Design review of the part built by this model. Coordinates are the model's own, in mm. Face numbers are marked on the shaded views. Give positions to 0.01 mm unless a question says otherwise; leave off trailing zeros. Loops run counter-clockwise (first coordinate to the right, second up) from the corner with the lowest first, then second, coordinate; pieces in that order, holes last.
Autodesk Inventor part; units mm, degrees
ref_plane "YZ Plane" through (0, 0, 0) normal (1, 0, 0) x (0, 1, 0)
ref_plane "XZ Plane" through (0, 0, 0) normal (0, 1, 0) x (-1, 0, 0)
ref_plane "XY Plane" through (0, 0, 0) normal (0, 0, 1) x (1, 0, 0)
sketch "Sketch1" plane through (0, 0, 0) normal (0, 0, 1) x (1, 0, 0)
  line L0 (0, 3) -> (3, 3)
  line L1 (6, 0) -> (6, 0)
  line L2 (3, -3) -> (0, -3)
  line L3 (0, -3) -> (0, 3)
  arc A0 (6, 0) -> (3, 3) centre (3, 0) ccw
  arc A1 (3, -3) -> (6, 0) centre (3, 0) ccw
  point P0 (0, 0)
  point P1 (0, 0)
  dimension "d0" = 3
  dimension "d1" = 6
  dimension "d2" = 6
extrude "Extrusion1" add sketch "Sketch1" along normal blind 6.5
sketch "Sketch2" plane through (0, -3, 0) normal (-1, 0, 0) x (0, 0, 1)
  line L0 (0, 6) -> (6.5, 6)
  line L1 (6.5, 6) -> (6.5, 0)
  line L2 (0, 0) -> (6.5, 0)
  line L3 (0, 0) -> (0, 6)
  line L4 (3.25, 6) -> (3.25, 0) construction
  line L5 (0, 3) -> (6.5, 3) construction
  point P0 (3.25, 3)
hole "Hole1" at (0, 0, 3.25) direction (1, 0, 0) diameter 3.2 depth 2
properties part number "Belt Tensioner" material "PC/ABS Plastic"
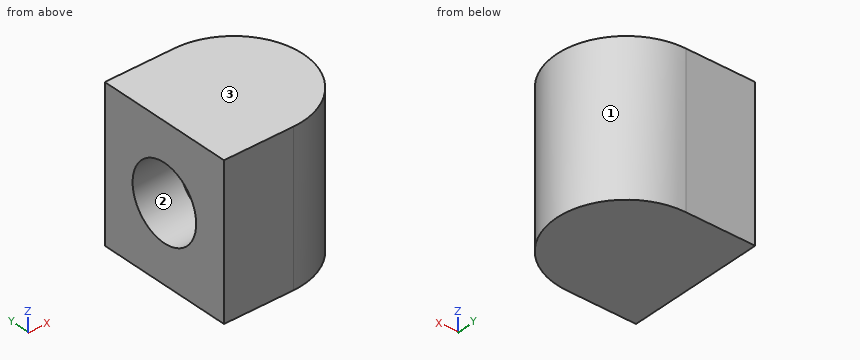
Q1. Take a section at B-B (z = 3.25). Give the boundary of the cut face in (x, y), plus the area to 3 significant figures.
Results:
outline: (0, -3) - (3, -3) arc R3 ccw to (3, 3) - (0, 3) - (0, 1.6) - (2, 1.6) - (2, -1.6) - (0, -1.6) - close
area: 25.7 mm2
Q2. Take a section at D-D (x = 3.9). Give the boundary of the cut face in (y, z).
Results:
outline: (-2.86, 0) - (2.86, 0) - (2.86, 6.5) - (-2.86, 6.5) - close
Q3. Draft analysis for pull direction Z (two halves, no side actions). For the marked faces 1, 2 and 3, state which applies: pulls with the +Z half, pulls with the -Z half, needs draft (parallel to the pull), parting line crosses it, or undercut.
Results:
face 1: needs draft
face 2: undercut
face 3: pulls with the +Z half
Q4. Take a section at C-C (y = 0). Give the boundary of the cut face in (x, z), plus the area to 3 significant figures.
Results:
outline: (0, 0) - (6, 0) - (6, 6.5) - (0, 6.5) - (0, 4.85) - (2, 4.85) - (2, 1.65) - (0, 1.65) - close
area: 32.6 mm2
Q5. Wall thickness on line 1 (Y direction, x = 1.55, z = 3.25); line 2 (Z direction, x = 1.55, y = 0); line 3 (Y direction, x = 1.6, z = 4.25): over which ranges is each line inside the solid? List them lowest first.
Results:
line 1: y = -3 to -1.6, 1.6 to 3
line 2: z = 0 to 1.65, 4.85 to 6.5
line 3: y = -3 to -1.25, 1.25 to 3
Q6. Insertion check: pin 1 (1 mm diameter, centred on x = 5.5, z = 5, fed in from -Y). The pin has a flat end and moves straight along its axis. Give the tip position at first contact, or say it passes through.
Results:
pin 1: stops at y = -2.24
Q7. Take a section at A-A (x = 1.85). Give the boundary of the cut face in (y, z).
Results:
outline: (-3, 0) - (3, 0) - (3, 6.5) - (-3, 6.5) - close; hole circle Ø3.2 at (0, 3.25)
